Could you check a few things on this model? Use its own coordinates, in mm. A direction names the side the tool comes from. Give positions to 0.01 mm unless a question says otherwise; leave off trailing zeros. Use a Markdown table: item, result. Add a question column.
1) If I drill on line 1 along Y through (x, z) = (0, -55.5); line 2 along X through (y, z) = (-6.75, 118); line 3 along X through (y, z) = (-5.75, -9), over which ranges is the centre line in solid material (lowest first)? Write a range as [from, to].
2) We'd pull the mould along Y, two halves only. Please class faces 1 (the flat face through (-3.901, 0, 2)), 2 (the flat face through (0, 3.901, 2)), 3 (the flat face through (0, -3.901, 2)): +Y half, -Y half, draft (parallel to the pull), parting line (faces both ways), or undercut.
3) Which directions (+Z, -Z, +X, -X, +Y, -Y) give clear straight access to the entire face, cutting with the end or side of a thin tool? Please do faces 4 (the flat face through (3.901, 0, 2)), 5 (the flat face through (-2.4, 0.1, -150)).
4) Will these pins go through, and if not, where does the flat tip stop? pin 1 Ø1 at (y, z) = (-0.5, 27.5) entering from +X; pin 2 Ø6 at (y, z) = (-0.5, 68) entering from -X; pin 3 Ø6 at (y, z) = (0.5, -66.5) entering from +X.
5) Suppose I cut it at A-A on z = 46.5. Count the separate pieces of the cut face and the enclosed holes in it, and give its area (3 significant figures).
```python
from build123d import *

# Parameters (mm, degrees)
ESQUISSE1_R        = 2.1
BOSS_EXTRU_2_DEPTH = 150


with BuildPart() as part:
    # Esquisse1 → Boss.-Extru.2 (new, symmetric)
    with BuildSketch(Plane.XY):
        with BuildLine():
            Line((-3.900660172, 0), (-3.900660172, -2.84))
            Line((-3.900660172, -2.84), (-6.56, -5.499339828))
            Line((-6.56, -5.499339828), (-8.2, -5.499339828))
            Line((-8.2, -5.499339828), (-8.2, -2.84))
            Line((-8.2, -2.84), (-10, -4.64))
            Line((-10, -4.64), (-10, -8.2))
            ThreePointArc((-10, -8.2), (-9.472792206, -9.472792206), (-8.2, -10))
            Line((-8.2, -10), (-4.64, -10))
            Line((-4.64, -10), (-2.84, -8.2))
            Line((-2.84, -8.2), (-5.499339828, -8.2))
            Line((-5.499339828, -8.2), (-5.499339828, -6.56))
            Line((-5.499339828, -6.56), (-2.84, -3.900660172))
            Line((-2.84, -3.900660172), (0, -3.900660172))
            Line((0, -3.900660172), (2.84, -3.900660172))
            Line((2.84, -3.900660172), (5.499339828, -6.56))
            Line((5.499339828, -6.56), (5.499339828, -8.2))
            Line((5.499339828, -8.2), (2.84, -8.2))
            Line((2.84, -8.2), (4.64, -10))
            Line((4.64, -10), (8.2, -10))
            ThreePointArc((8.2, -10), (9.472792206, -9.472792206), (10, -8.2))
            Line((10, -8.2), (10, -4.64))
            Line((10, -4.64), (8.2, -2.84))
            Line((8.2, -2.84), (8.2, -5.499339828))
            Line((8.2, -5.499339828), (6.56, -5.499339828))
            Line((6.56, -5.499339828), (3.900660172, -2.84))
            Line((3.900660172, -2.84), (3.900660172, 0))
            Line((3.900660172, 0), (3.900660172, 2.84))
            Line((3.900660172, 2.84), (6.56, 5.499339828))
            Line((6.56, 5.499339828), (8.2, 5.499339828))
            Line((8.2, 5.499339828), (8.2, 2.84))
            Line((8.2, 2.84), (10, 4.64))
            Line((10, 4.64), (10, 8.2))
            ThreePointArc((10, 8.2), (9.472792206, 9.472792206), (8.2, 10))
            Line((8.2, 10), (4.64, 10))
            Line((4.64, 10), (2.84, 8.2))
            Line((2.84, 8.2), (5.499339828, 8.2))
            Line((5.499339828, 8.2), (5.499339828, 6.56))
            Line((5.499339828, 6.56), (2.84, 3.900660172))
            Line((2.84, 3.900660172), (0, 3.900660172))
            Line((0, 3.900660172), (-2.84, 3.900660172))
            Line((-2.84, 3.900660172), (-5.499339828, 6.56))
            Line((-5.499339828, 6.56), (-5.499339828, 8.2))
            Line((-5.499339828, 8.2), (-2.84, 8.2))
            Line((-2.84, 8.2), (-4.64, 10))
            Line((-4.64, 10), (-8.2, 10))
            ThreePointArc((-8.2, 10), (-9.472792206, 9.472792206), (-10, 8.2))
            Line((-10, 8.2), (-10, 4.64))
            Line((-10, 4.64), (-8.2, 2.84))
            Line((-8.2, 2.84), (-8.2, 5.499339828))
            Line((-8.2, 5.499339828), (-6.56, 5.499339828))
            Line((-6.56, 5.499339828), (-3.900660172, 2.84))
            Line((-3.900660172, 2.84), (-3.900660172, 0))
        make_face()
        Circle(ESQUISSE1_R, mode=Mode.SUBTRACT)
        Polygon((-8.2, -8.2), (-8.2, -6.569339828), (-7.63, -6.569339828), (-6.569339828, -7.63), (-6.569339828, -8.2), align=None, mode=Mode.SUBTRACT)
        Polygon((-8.2, 6.569339828), (-8.2, 8.2), (-6.569339828, 8.2), (-6.569339828, 7.63), (-7.63, 6.569339828), align=None, mode=Mode.SUBTRACT)
        Polygon((6.569339828, 8.2), (8.2, 8.2), (8.2, 6.569339828), (7.63, 6.569339828), (6.569339828, 7.63), align=None, mode=Mode.SUBTRACT)
        Polygon((8.2, -6.569339828), (8.2, -8.2), (6.569339828, -8.2), (6.569339828, -7.63), (7.63, -6.569339828), align=None, mode=Mode.SUBTRACT)
    extrude(amount=BOSS_EXTRU_2_DEPTH, both=True)


solid = part.part
```
Answer block:
| question | item | result |
|---|---|---|
| 1 | line 1 | y = [-3.9, -2.1], [2.1, 3.9] |
| 1 | line 2 | x = [-10, -8.2], [-7.45, -5.5], [5.5, 7.45], [8.2, 10] |
| 1 | line 3 | x = [-10, -4.69], [4.69, 10] |
| 2 | face 1 | undercut |
| 2 | face 2 | +Y half |
| 2 | face 3 | -Y half |
| 3 | face 4 | +Z, -Z, +X |
| 3 | face 5 | -Z, +X, -X, +Y, -Y |
| 4 | pin 1 | stops at x = 3.9 |
| 4 | pin 2 | stops at x = -8.86 |
| 4 | pin 3 | stops at x = 8.86 |
| 5 | separate pieces | 1 |
| 5 | enclosed holes | 5 |
| 5 | area | 160 mm^2 |
